from build123d import *

# Parameters (mm, degrees)
CYLINDER003_R     = 4
CYLINDER003_DEPTH = 10
CYLINDER002_R     = 3
CYLINDER002_DEPTH = 3
CYLINDER001_R     = 10
CYLINDER001_DEPTH = 10
CYLINDER_R        = 12
CYLINDER_DEPTH    = 3


with BuildPart() as cilindro003:
    # Cylinder003 → Cylinder003 (new body)
    with BuildSketch(Plane(origin=(3.2, 1.8, 0), x_dir=(1, 0, 0), z_dir=(0, 0, 1))):
        Circle(CYLINDER003_R)
    extrude(amount=CYLINDER003_DEPTH)


with BuildPart() as cut001:
    # Cylinder002 → Cylinder002 (new body)
    with BuildSketch(Plane.XY):
        Circle(CYLINDER002_R)
    extrude(amount=CYLINDER002_DEPTH)

    # Cut001: cut Cilindro003
    add(cilindro003.part, mode=Mode.SUBTRACT)


with BuildPart() as cut001_1:
    # Cut001 placement: moved
    add(cut001.part.moved(Location((-9, 10.2, 0))))


with BuildPart() as fusion:
    # Part__Mirroring: instance of Cut001
    add(cut001_1.part.mirror(Plane(origin=(0, 0, 0), x_dir=(0, -1, 0), z_dir=(1, 0, 0))))

    # Fusion: union Cut001
    add(cut001_1.part)


with BuildPart() as cilindro001:
    # Cylinder001 → Cylinder001 (new body)
    with BuildSketch(Plane.XY.offset(-4)):
        Circle(CYLINDER001_R)
    extrude(amount=CYLINDER001_DEPTH)


with BuildPart() as fusion001:
    # Cylinder → Cylinder (new body)
    with BuildSketch(Plane.XY):
        Circle(CYLINDER_R)
    extrude(amount=CYLINDER_DEPTH)

    # Cut: cut Cilindro001
    add(cilindro001.part, mode=Mode.SUBTRACT)

    # Fusion001: union Fusion
    add(fusion.part)


solid = fusion001.part
Geometry check sheet. Reference: the model listing, model coordinates, mm. A direction names the side the tool comes from. Give positions to 0.01 mm unless a question says otherwise; leave off trailing zeros. Write each loop counter-clockwise with the first axis right and the second up, starting at its lowest first coordinate (ties: lowest second). Pieces come first, ordered by that corner, then holes. Notation, with made-up numbers: M -32.75,48 L -16.75,48 A27 cw -16.75,75 Z; hole C -38,7.25 d3. An arc over 180 degrees is marked long. Answer as CSV lines item,"result". Start each with the question number.
Q1. Section check C-C, the plane y = 11.25. Record the cut outline in (x, z).
Q2. Release check for a two-part mould opening along Y. For faces 3 (the face through (2, 10, 3)), 4 (the face through (0, -12, 1)), 5 (the face through (0, 12, 1)) record: pulls with the +Y half, pulls with the -Y half, needs draft (parallel to the pull), parting line crosses it, or undercut.
Q3. Material ranges on L1, parallel to X at y = 0, z = 1.75; L2, parallel to X at y = 11, z = 2; L3, parallel to Y at x = -0.75, z = 2.55, recorded low to high.
Q4. Tool access check on faces 1 (the face through (2, 10, 0)), 2 (the face through (-9.603, 10.76, 1.479)). Record the directions out of +Z, -Z, +X, -X, +Y, -Y that give a thin tool (end or side, any length) a straight path to the whole face; none if there is none.
Q5. Section check D-D, the plane z = 1.75. Record the cut outline in (x, y), then the cut area to 3 significant figures.
Q6. Section check A-A, the plane x = 0. Record the cut outline in (y, z), then the cut area to 3 significant figures.
Q7. Go/stop test with a flat-tipped pin: pin 1 (1 mm diameter, centred on x = -8, z = 1.5, fed in from -Y). Record where the tip stops, or that it passes through.
Geometry says:
1,outline,"M -11.81,0 L -9.73,0 L -9.73,3 L -11.81,3 Z; M -4.18,0 L 4.18,0 L 4.18,3 L -4.18,3 Z; M 9.73,0 L 11.81,0 L 11.81,3 L 9.73,3 Z"
2,face 3,"needs draft"
2,face 4,"undercut"
2,face 5,"pulls with the +Y half"
3,L1,"-12 to -10, 10 to 12"
3,L2,"-11.89 to -9.67, -4.8 to 4.8, 9.67 to 11.89"
3,L3,"-11.98 to -9.97, 9.97 to 11.98"
4,face 1,"-Z, +X, -X, +Y, -Y"
4,face 2,"+Z, -Z"
5,outline,"M -9.64,13.13 A3 ccw -9.56,7.25 A12 ccw long 9.56,7.25 A3 ccw 9.64,13.13 A4 cw 8.18,8.78 A12 ccw -8.18,8.78 A4 cw Z; hole C 0,0 d20"
5,area,"163 mm^2"
6,outline,"M -12,0 L -10,0 L -10,3 L -12,3 Z; M 10,0 L 12,0 L 12,3 L 10,3 Z"
6,area,"12.0 mm^2"
7,pin 1,"y = -9.37"
